Geometry: final body of the model. Coordinates: model frame, mm. Face numbers are marked on the shaded views. A direction names the side the tool comes from. Give positions to 0.01 mm unless a question says otherwise; leave off trailing zeros. Order: outer loops, then holes, each group sorted by start corner. A loop starts at its lowest first (then second) coordinate and runs counter-clockwise, first axis right, second up. Notation, with made-up numbers: (-1, 11.5) - (8, 11.5) arc R17 ccw to (8, 17.5) - close; hole circle Ø2 at (-13.5, -33). An arc over 180 degrees is marked (long way). One line per item, written item: value.
```python
from build123d import *

# Parameters (mm, degrees)
SKETCH1_W                                    = 48
SKETCH1_H                                    = 48
SKETCH1_W_2                                  = 42
SKETCH1_H_2                                  = 42
BOSS_EXTRUDE1_DEPTH                          = 65
SKETCH3_W                                    = 75
SKETCH3_H                                    = 75
BOSS_EXTRUDE2_DEPTH                          = 5
SKETCH8_W                                    = 75
SKETCH8_H                                    = 75
SKETCH8_W_2                                  = 42
SKETCH8_H_2                                  = 42
BOSS_EXTRUDE3_DEPTH                          = 5.047079132
FILLET1_R                                    = 2
CBORE_FOR_M6_HEX_SOCKET_HEAD_CAP_SCR_2_COUNT = 2
CBORE_FOR_M6_HEX_SOCKET_HEAD_CAP_SCR_2_PITCH = 50
CBORE_FOR_M6_HEX_SOCKET_HEAD_CAP_SCR_3_COUNT = 2
CBORE_FOR_M6_HEX_SOCKET_HEAD_CAP_SCR_3_PITCH = 61.5
CBORE_FOR_M6_HEX_SOCKET_HEAD_CAP_SCR_4_COUNT = 2
CBORE_FOR_M6_HEX_SOCKET_HEAD_CAP_SCR_4_PITCH = 79.260645973
FILLET2_R                                    = 1
CHAMFER1_SIZE                                = 2


with BuildPart() as part:
    # Sketch1 → Boss-Extrude1 (new body)
    with BuildSketch(Plane(origin=(0, 0, 0), x_dir=(0, 1, 0), z_dir=(0, 0, 1))):
        with Locations((-1.048003873, 6.146094376)):
            Rectangle(SKETCH1_W, SKETCH1_H)
        with Locations((-1.048003873, 6.146094376)):
            Rectangle(SKETCH1_W_2, SKETCH1_H_2, mode=Mode.SUBTRACT)
    extrude(amount=BOSS_EXTRUDE1_DEPTH)

    # Sketch3 → Boss-Extrude2 (add)
    with BuildSketch(Plane(origin=(0, 0, 0), x_dir=(1, 0, 0), z_dir=(0, 0, -1))):
        with Locations((-6.146094376, 1.048003873)):
            Rectangle(SKETCH3_W, SKETCH3_H)
    extrude(amount=BOSS_EXTRUDE2_DEPTH)

    # Sketch8 → Boss-Extrude3 (add)
    with BuildSketch(Plane.XY):
        with Locations((-6.146094376, -1.048003873)):
            Rectangle(SKETCH8_W, SKETCH8_H)
        with Locations((-6.146094376, -1.048003873)):
            Rectangle(SKETCH8_W_2, SKETCH8_H_2, mode=Mode.SUBTRACT)
    extrude(amount=BOSS_EXTRUDE3_DEPTH)

    # Fillet1
    fillet1_edges = [part.edges().sort_by_distance(p)[0] for p in [
        (17.853905624, 22.951996127, 35.023539566),
        (17.853905624, -25.048003873, 35.023539566),
        (-30.146094376, -25.048003873, 35.023539566),
        (-30.146094376, 22.951996127, 35.023539566),
        (-43.646094376, -38.548003873, 0.023539566),
        (31.353905624, -38.548003873, 0.023539566),
        (31.353905624, 36.451996127, 0.023539566),
        (-43.646094376, 36.451996127, 0.023539566),
    ]]
    fillet(fillet1_edges, radius=FILLET1_R)

    # Sketch15 → CBORE for M6 Hex Socket Head Cap Screw2 (revolve, cut)
    with BuildSketch(Plane(origin=(-36.896094376, 23.951996127, 5.047079132), x_dir=(0, -1, 0), z_dir=(1, 0, 0))):
        Polygon((0, 0), (0, 10.047079132), (3.3, 10.047079132), (3.3, 6.4), (5.5, 6.4), (5.5, 0.025), (5.525, 0), align=None)
    cbore_for_m6_hex_socket_head_cap_screw2 = revolve(axis=Axis((-36.896094376, 23.951996127, 11.397079132), (0, 0, -1)), mode=Mode.SUBTRACT)

    # CBORE for M6 Hex Socket Head Cap Scr 2: CBORE for M6 Hex Socket Head Cap Screw2 ×2
    with Locations(*[(0, -i * CBORE_FOR_M6_HEX_SOCKET_HEAD_CAP_SCR_2_PITCH, 0) for i in range(1, CBORE_FOR_M6_HEX_SOCKET_HEAD_CAP_SCR_2_COUNT)]):
        add(cbore_for_m6_hex_socket_head_cap_screw2, mode=Mode.SUBTRACT)

    # CBORE for M6 Hex Socket Head Cap Scr 3: CBORE for M6 Hex Socket Head Cap Screw2 ×2
    with Locations(*[(i * CBORE_FOR_M6_HEX_SOCKET_HEAD_CAP_SCR_3_PITCH, 0, 0) for i in range(1, CBORE_FOR_M6_HEX_SOCKET_HEAD_CAP_SCR_3_COUNT)]):
        add(cbore_for_m6_hex_socket_head_cap_screw2, mode=Mode.SUBTRACT)

    # CBORE for M6 Hex Socket Head Cap Scr 4: CBORE for M6 Hex Socket Head Cap Screw2 ×2
    with Locations(*[Vector(0.7759210039901774, -0.63083008454486, 0) * (i * CBORE_FOR_M6_HEX_SOCKET_HEAD_CAP_SCR_4_PITCH) for i in range(1, CBORE_FOR_M6_HEX_SOCKET_HEAD_CAP_SCR_4_COUNT)]):
        add(cbore_for_m6_hex_socket_head_cap_screw2, mode=Mode.SUBTRACT)

    # Fillet2
    fillet2_edges = [part.edges().sort_by_distance(p)[0] for p in [
        (14.853905624, -22.048003873, 32.5),
        (14.853905624, 19.951996127, 32.5),
        (-27.146094376, 19.951996127, 32.5),
        (-27.146094376, -22.048003873, 32.5),
    ]]
    fillet(fillet2_edges, radius=FILLET2_R)

    # Chamfer1
    chamfer1_edges = [part.edges().sort_by_distance(p)[0] for p in [
        (-6.146094376, 36.451996127, -5),
        (-6.146094376, -38.548003873, -5),
        (-43.646094376, -1.048003873, -5),
        (30.768119187, -37.962217436, -5),
        (-43.060307938, -37.962217436, -5),
        (-43.060307938, 35.866209689, -5),
        (30.768119187, 35.866209689, -5),
        (31.353905624, -1.048003873, -5),
    ]]
    chamfer(chamfer1_edges, length=CHAMFER1_SIZE)


solid = part.part
```
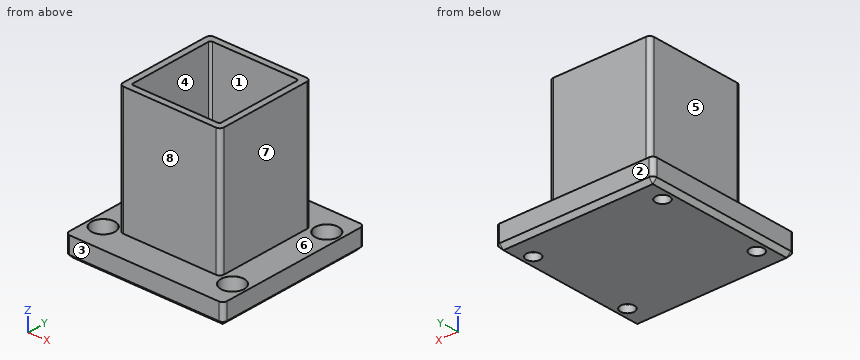
1) Section D-D, the plane z = 2. Return loops of the section in (x, y).
Answers below:
outline: (-43.65, -36.55) arc R2 ccw to (-41.65, -38.55) - (29.35, -38.55) arc R2 ccw to (31.35, -36.55) - (31.35, 34.45) arc R2 ccw to (29.35, 36.45) - (-41.65, 36.45) arc R2 ccw to (-43.65, 34.45) - close; hole circle Ø11 at (-36.9, -26.05); hole circle Ø11 at (-36.9, 23.95); hole (-27.15, -21.05) arc R1 ccw to (-26.15, -22.05) - (13.85, -22.05) arc R1 ccw to (14.85, -21.05) - (14.85, 18.95) arc R1 ccw to (13.85, 19.95) - (-26.15, 19.95) arc R1 ccw to (-27.15, 18.95) - close; hole circle Ø11 at (24.6, -26.05); hole circle Ø11 at (24.6, 23.95)
2) Material intervals for line 1 along X through (y, z) = (-1, 53); line 2 along Y through (x, z) = (11, 53.5); line 3 along X through (y, z) = (17, 2.5), sorted ascending.
Answers below:
line 1: -30.15 to -27.15, 14.85 to 17.85
line 2: -25.05 to -22.05, 19.95 to 22.95
line 3: -43.65 to -27.15, 14.85 to 31.35
3) Section C-C, the plane x = 0. Return loops of the section in (y, z), then the cut area to 3 significant figures.
Answers below:
outline: (-38.55, -3) - (-36.55, -5) - (34.45, -5) - (36.45, -3) - (36.45, 5.05) - (22.95, 5.05) - (22.95, 65) - (19.95, 65) - (19.95, 0) - (-22.05, 0) - (-22.05, 65) - (-25.05, 65) - (-25.05, 5.05) - (-38.55, 5.05) - close
area: 897 mm^2
4) First-contact query: pin 1 (20 mm diameter, centred on x = 2.5, z = 41.5, fed in from -Y); pin 2 (3.5 mm diameter, centred on x = -36, y = -28, fed in from +Z); pin 3 (20 mm diameter, centred on y = -3.5, z = 46, fed in from +X). Flat tips, straight axial feed; report the tip coordinate or a pass-through.
Answers below:
pin 1: y = -25.05
pin 2: z = -1.35
pin 3: x = 17.85
5) Section A-A, the plane z = 30. Return loops of the section in (x, y).
Answers below:
outline: (-30.15, -23.05) arc R2 ccw to (-28.15, -25.05) - (15.85, -25.05) arc R2 ccw to (17.85, -23.05) - (17.85, 20.95) arc R2 ccw to (15.85, 22.95) - (-28.15, 22.95) arc R2 ccw to (-30.15, 20.95) - close; hole (-27.15, -21.05) arc R1 ccw to (-26.15, -22.05) - (13.85, -22.05) arc R1 ccw to (14.85, -21.05) - (14.85, 18.95) arc R1 ccw to (13.85, 19.95) - (-26.15, 19.95) arc R1 ccw to (-27.15, 18.95) - close
6) Mould query, pull axis Y, two halves, no side actions, for the marked faces 1, 2, 3 and 4. Classes: released by +Y, released by -Y, zero draft, split by the parting line, or undercut.
Answers below:
face 1: undercut
face 2: released by +Y
face 3: released by -Y
face 4: undercut
7) Set-up query: the marked faces 5, 6, 7 and 8. Return all of +Z, -Z, +X, -X, +Y, -Y with unobstructed straight access to the full face (end or side cutting, diameter ignored); none if empty.
Answers below:
face 5: +Z, -X, +Y, -Y
face 6: +Z
face 7: +Z, +X, +Y, -Y
face 8: +Z, +X, -X, -Y
8) Section B-B, the plane y = -14. Return loops of the section in (x, z).
Answers below:
outline: (-43.65, -3) - (-41.65, -5) - (29.35, -5) - (31.35, -3) - (31.35, 5.05) - (17.85, 5.05) - (17.85, 65) - (14.85, 65) - (14.85, 0) - (-27.15, 0) - (-27.15, 65) - (-30.15, 65) - (-30.15, 5.05) - (-43.65, 5.05) - close
